Model file for the job. Use its own axes, mm. A direction names the side the tool comes from. Round coordinates to 2 decimals unless told otherwise and drop trailing zeros. Order: outer loops, then holes, each group sorted by start corner. A loop starts at its lowest first (then second) coordinate and runs counter-clockwise, first axis right, second up. Notation, with made-up numbers: (-19.75, 69.25) - (32.25, 69.25) arc R15 ccw to (32.25, 88.25) - close; hole circle Ø1 at (-13.5, -35). An arc over 180 degrees is marked (long way). Put each result on its own line as item: value. Start each with the question number.
Item 1: Pin check, flat tips, straight feed: pin 1 Ø2 at (x, z) = (-20, -11.49) entering from -Y; pin 2 Ø6 at (x, z) = (-11, 7.5) entering from +Y. Stop position of each tip, or through.
Item 2: Saw through at D-D on y = 4.75. List the corners of the cut face in (x, z).
Item 3: Saw through at A-A on x = -20. List the corners of the cut face in (y, z), plus the area to 3 significant figures.
Item 4: Which spindle directions (+Z, -Z, +X, -X, +Y, -Y) get a long thin tool onto all of the face, cutting with end or side? Do faces 4 (the face through (16.365, 5.828, -0.172)), 5 (the face through (20, 13.461, -10)), 6 (the face through (-2, 2, 15)), 7 (the face through (-16, 5, 0)), 8 (the face through (7, 1.5, 7.4)). Say none if no direction does.
Item 5: Probe probe 1 along Z at (x, y) = (0, 0.6); probe 2 along X at (y, z) = (2.35, 7.5); probe 3 along X at (y, z) = (4, -7). List the from-to ranges inside material, lowest first.
Item 6: Saw through at C-C on x = 12. List the corners of the cut face in (y, z), plus the area to 3 significant figures.
Item 7: Mould opens along Z. For faces 1 (the face through (16, 5, 0)), 2 (the face through (-2, 2, -15)), 3 (the face through (7, 1.5, -7.6)) say: pulls with the +Z half, pulls with the -Z half, needs draft (parallel to the pull), parting line crosses it, or undercut.
Item 8: Saw through at B-B on z = 0. List the corners of the cut face in (x, y), plus the area to 3 significant figures.
```python
from build123d import *

# Parameters (mm, degrees)
SKETCH2_W                = 32
SKETCH2_H                = 30
BOSS_EXTRUDE1_DEPTH      = 2.922658801
BOSS_EXTRUDE2_DEPTH      = 25
BOSS_EXTRUDE2_DEPTH_BACK = 2.922659
SKETCH3_W                = 8
SKETCH3_H                = 30
CUT_EXTRUDE1_DEPTH       = 58.521082001
CUT_EXTRUDE1_DEPTH_BACK  = 58.521082001
SKETCH4_R                = 8
M3X0_5_TAPPED_HOLE1_D    = 2.5
SKETCH7_R                = 2.5
CUT_EXTRUDE2_DEPTH       = 38.762415177
SKETCH8_W                = 30
SKETCH8_H                = 18.9613294
CUT_EXTRUDE3_DEPTH       = 58.521082001
SKETCH9_W                = 30
SKETCH9_H                = 0.5
CUT_EXTRUDE4_DEPTH       = 53.19117472
M3X0_5_TAPPED_HOLE2_D    = 2.5
CHAMFER1_SIZE            = 0.5


with BuildPart() as part:
    # Sketch2 → Boss-Extrude1 (new body)
    with BuildSketch(Plane(origin=(0, 0, 0), x_dir=(1, 0, 0), z_dir=(0, 1, 0))):
        Rectangle(SKETCH2_W, SKETCH2_H)
    extrude(amount=BOSS_EXTRUDE1_DEPTH)

    # Sketch3 → Boss-Extrude2 (add, two sides: drawn at the far end of the back side and taken through both)
    with BuildSketch(Plane(origin=(0, 2.922658801, 0), x_dir=(1, 0, 0), z_dir=(0, 1, 0)).offset(-BOSS_EXTRUDE2_DEPTH_BACK)):
        with Locations((-20, 0)):
            Rectangle(SKETCH3_W, SKETCH3_H)
        with Locations((20, 0)):
            Rectangle(SKETCH3_W, SKETCH3_H)
    extrude(amount=BOSS_EXTRUDE2_DEPTH + BOSS_EXTRUDE2_DEPTH_BACK)

    # Sketch4 → Cut-Extrude1 (cut, two sides: drawn at the far end of the back side and taken through both)
    with BuildSketch(Plane(origin=(24, 0, 0), x_dir=(0, 0, -1), z_dir=(1, 0, 0)).offset(-CUT_EXTRUDE1_DEPTH_BACK)):
        with Locations((0, 13.961329401)):
            Circle(SKETCH4_R)
    extrude(amount=CUT_EXTRUDE1_DEPTH + CUT_EXTRUDE1_DEPTH_BACK, mode=Mode.SUBTRACT)

    # M3x0.5 Tapped Hole1 (through all)
    with Locations(Plane(origin=(0, 2.922658801, 0), x_dir=(1, 0, 0), z_dir=(0, 1, 0))):
        with Locations((12, 0), (0, 0), (-12, 0)):
            Hole(M3X0_5_TAPPED_HOLE1_D / 2)

    # Sketch7 → Cut-Extrude2 (cut, through all)
    with BuildSketch(Plane(origin=(0, 2.922658801, 0), x_dir=(1, 0, 0), z_dir=(0, 1, 0))):
        with Locations(Location((-11, 7.5, 0), (0, 0, 270))):
            Circle(SKETCH7_R)
        with Locations(Location((-11, -7.5, 0), (0, 0, 270))):
            Circle(SKETCH7_R)
        with Locations(Location((11, -7.5, 0), (0, 0, 270))):
            Circle(SKETCH7_R)
        with Locations(Location((11, 7.5, 0), (0, 0, 270))):
            Circle(SKETCH7_R)
        with BuildLine():
            Line((-3, 11.5), (3, 11.5))
            ThreePointArc((3, 11.5), (7, 7.5), (3, 3.5))
            Line((3, 3.5), (-3, 3.5))
            ThreePointArc((-3, 3.5), (-7, 7.5), (-3, 11.5))
        make_face()
        with BuildLine():
            Line((-3, -3.5), (3, -3.5))
            ThreePointArc((3, -3.5), (7, -7.5), (3, -11.5))
            Line((3, -11.5), (-3, -11.5))
            ThreePointArc((-3, -11.5), (-7, -7.5), (-3, -3.5))
        make_face()
    extrude(amount=-CUT_EXTRUDE2_DEPTH, mode=Mode.SUBTRACT)

    # Sketch8 → Cut-Extrude3 (cut, through all)
    with BuildSketch(Plane(origin=(24, 0, 0), x_dir=(0, 0, -1), z_dir=(1, 0, 0))):
        with Locations((0, 23.441994101)):
            Rectangle(SKETCH8_W, SKETCH8_H)
    extrude(amount=-CUT_EXTRUDE3_DEPTH, mode=Mode.SUBTRACT)

    # Sketch9 → Cut-Extrude4 (cut, through all)
    with BuildSketch(Plane(origin=(24, 0, 0), x_dir=(0, 0, -1), z_dir=(1, 0, 0))):
        with Locations((0, 13.711329401)):
            Rectangle(SKETCH9_W, SKETCH9_H)
    extrude(amount=-CUT_EXTRUDE4_DEPTH, mode=Mode.SUBTRACT)

    # M3x0.5 Tapped Hole2 (through all)
    with Locations(Plane(origin=(0, 13.461329401, 0), x_dir=(1, 0, 0), z_dir=(0, 1, 0))):
        with Locations((-20, 11.492179856), (20, -11.492179856), (20, 11.492179856), (-20, -11.492179856)):
            Hole(M3X0_5_TAPPED_HOLE2_D / 2)

    # Chamfer1
    chamfer1_edges = [part.edges().sort_by_distance(p)[0] for p in [
        (-16, 8.191994101, -15),
        (-16, 8.191994101, 15),
        (-24, 6.730664601, 15),
        (-24, 6.730664601, -15),
        (-24, -1.99e-07, 0),
        (-16, 5.961329401, 0),
        (-24, 5.961329401, 0),
        (24, 5.961329401, 0),
        (16, 5.961329401, 0),
        (0, 2.922658801, -15),
        (16, 8.191994101, 15),
        (16, 8.191994101, -15),
        (24, 6.730664601, -15),
        (24, 6.730664601, 15),
        (24, -1.99e-07, 0),
        (0, 0, -15),
        (0, 0, 15),
        (0, 2.922658801, 15),
    ]]
    chamfer(chamfer1_edges, length=CHAMFER1_SIZE)


solid = part.part
```
Results found:
1. pin 1: passes through
1. pin 2: stops at y = 2.92
2. outline: (-24, -14.5) - (-23.5, -15) - (-16.5, -15) - (-16, -14.5) - (-16, 14.5) - (-16.5, 15) - (-23.5, 15) - (-24, 14.5) - close; (16, -14.5) - (16.5, -15) - (23.5, -15) - (24, -14.5) - (24, 14.5) - (23.5, 15) - (16.5, 15) - (16, 14.5) - close; hole circle Ø2.5 at (-20, -11.49); hole circle Ø2.5 at (-20, 11.49); hole circle Ø2.5 at (20, -11.49); hole circle Ø2.5 at (20, 11.49)
3. outline: (0, -14.5) - (0.5, -15) - (13.46, -15) - (13.46, -12.74) - (0, -12.74) - close; (0, -10.24) - (13.46, -10.24) - (13.46, -7.98) arc R8 cw to (13.46, 7.98) - (13.46, 10.24) - (0, 10.24) - close; (0, 12.74) - (13.46, 12.74) - (13.46, 15) - (0.5, 15) - (0, 14.5) - close
3. area: 244 mm²
4. face 4: +Y
4. face 5: +Z, -Z, +X, -X, +Y
4. face 6: +Z, +X, -X, +Y, -Y
4. face 7: +Z, -Z, +Y
4. face 8: +Y, -Y
5. probe 1: z = -15 to -11.5, -3.5 to -1.25, 1.25 to 3.5, 11.5 to 15
5. probe 2: x = -24 to -13.5, -8.5 to -7, 7 to 8.5, 13.5 to 24
5. probe 3: x = -24 to -16, 16 to 24
6. outline: (0, -14.5) - (0.5, -15) - (2.42, -15) - (2.92, -14.5) - (2.92, -9.79) - (0, -9.79) - close; (0, -5.21) - (2.92, -5.21) - (2.92, -1.25) - (0, -1.25) - close; (0, 1.25) - (2.92, 1.25) - (2.92, 5.21) - (0, 5.21) - close; (0, 9.79) - (2.92, 9.79) - (2.92, 14.5) - (2.42, 15) - (0.5, 15) - (0, 14.5) - close
6. area: 53.1 mm²
7. face 1: needs draft
7. face 2: pulls with the -Z half
7. face 3: undercut
8. outline: (-24, 0.5) - (-23.5, 0) - (-13.25, 0) - (-13.25, 2.92) - (-16, 2.92) - (-16, 5.46) - (-16.5, 5.96) - (-23.5, 5.96) - (-24, 5.46) - close; (-10.75, 0) - (-1.25, 0) - (-1.25, 2.92) - (-10.75, 2.92) - close; (1.25, 0) - (10.75, 0) - (10.75, 2.92) - (1.25, 2.92) - close; (13.25, 0) - (23.5, 0) - (24, 0.5) - (24, 5.46) - (23.5, 5.96) - (16.5, 5.96) - (16, 5.46) - (16, 2.92) - (13.25, 2.92) - close
8. area: 166 mm²
